```python
from build123d import *

# Parameters (mm, degrees)
EXTRUDE_1_DEPTH     = 22.5
SKETCH_2_R          = 8
CUT_EXTRUDE_1_DEPTH = 10
CUT_EXTRUDE_2_REACH = 62.26
SKETCH_3_R          = 5


with BuildPart() as part:
    # Эскиз1 → Бобышка-Вытянуть1 (new, symmetric)
    with BuildSketch(Plane(origin=(0, 0, 0), x_dir=(1, 0, 0), z_dir=(0, 1, 0))):
        Polygon((50, 0), (-50, 0), (-50, 30), (-20, 30), (-20, 45), (-8, 45), (-5, 42), (-5, 10), (5, 10), (5, 42), (8, 45), (20, 45), (20, 30), (50, 30), align=None)
    extrude(amount=EXTRUDE_1_DEPTH, both=True)

    # Эскиз2 → Вырез-Вытянуть1 (cut)
    with BuildSketch(Plane(origin=(0, 0, -30), x_dir=(-1, 0, 0), z_dir=(0, 0, -1))):
        with Locations((37.5, 0)):
            Circle(SKETCH_2_R)
    cut_extrude_1 = extrude(amount=-CUT_EXTRUDE_1_DEPTH, mode=Mode.SUBTRACT)

    # Эскиз3 → Вырез-Вытянуть2 (cut, up to next)
    with BuildSketch(Plane(origin=(0, 0, -20), x_dir=(-1, 0, 0), z_dir=(0, 0, -1)), mode=Mode.PRIVATE) as cut_extrude_2_sk1:
        with Locations((37.5, 0)):
            Circle(SKETCH_3_R)
    cut_extrude_2_tool1 = extrude(cut_extrude_2_sk1.sketch, amount=-CUT_EXTRUDE_2_REACH, mode=Mode.PRIVATE) & part.part
    cut_extrude_2 = cut_extrude_2_tool1.solids().sort_by_distance((-37.5, 0, -20))[0]
    add(cut_extrude_2, mode=Mode.SUBTRACT)

    # Зеркальное отражение1: Вырез-Вытянуть1, Вырез-Вытянуть2 across plane
    add(cut_extrude_1.mirror(Plane(origin=(0, 0, 0), x_dir=(0, 0, 1), z_dir=(1, 0, 0))), mode=Mode.SUBTRACT)
    add(cut_extrude_2.mirror(Plane(origin=(0, 0, 0), x_dir=(0, 0, 1), z_dir=(1, 0, 0))), mode=Mode.SUBTRACT)


solid = part.part
```
Source: CAD feature listing. Evaluate the final solid. Frame: model axes, mm. A direction names the side the tool comes from. Give positions to 0.01 mm unless a question says otherwise; leave off trailing zeros. Write each loop counter-clockwise with the first axis right and the second up, starting at its lowest first coordinate (ties: lowest second). Pieces come first, ordered by that corner, then holes.
1. Section query C-C (x = 37.5). Return the cut outline in (y, z), then the cut area to 3 significant figures.
2. Access query for faces 5 (the face through (6, 0, -43)), 6 (the face through (-29, 0, -30)), 7 (the face through (20, 0, -38)). Directions: +Z, -Z, +X, -X, +Y, -Y. A direction counts if a zero-diameter tool reaches every point of the face in a straight line with its end or side. Return the directions, or none.
3. Pull-direction query (Y, two-part tool) for faces 1 (the face through (41, 4, -20)), 2 (the face through (-50, 0, -15)), 3 (the face through (1, 22.5, -8)), 4 (the face through (31.151, -4.868, -25.07)); classes: +Y half, -Y half, draft (parallel to the pull), parting line (faces both ways), or undercut.
4. Section query D-D (z = -28.5). Return the cut outline in (x, y).
5. Section query A-A (z = -12). Return the cut outline in (x, y).
6. Section query B-B (y = 0). Count the separate pieces of the cut face and the enclosed holes in it, then the cut area to 3 significant figures.
7. First-contact query: pin 1 (17.5 mm diameter, centred on x = -37, y = 1.5, fed in from -Z); pin 2 (8 mm diameter, centred on x = 0, y = 8, fed in from -Z); pin 3 (7.5 mm diameter, centred on y = 10, z = -35.5, fed in from -X). Flat tips, straight axial feed; report the tip coordinate or a pass-through.
8. Material intervals for line 1 along X through (y, z) = (14.5, -14.5); line 2 along Y through (x, z) = (37, -23); line 3 along Y through (x, z) = (37.5, -8.5), sorted ascending.
Output values:
1. outline: (-22.5, -30) - (-8, -30) - (-8, -20) - (-5, -20) - (-5, 0) - (-22.5, 0) - close; (5, -20) - (8, -20) - (8, -30) - (22.5, -30) - (22.5, 0) - (5, 0) - close
1. area: 990 mm2
2. face 5: -Z, +Y, -Y
2. face 6: -Z, -X, +Y, -Y
2. face 7: -Z, +X, +Y, -Y
3. face 1: undercut
3. face 2: draft
3. face 3: +Y half
3. face 4: undercut
4. outline: (-50, -22.5) - (-5, -22.5) - (-5, 22.5) - (-50, 22.5) - close; (5, -22.5) - (50, -22.5) - (50, 22.5) - (5, 22.5) - close; hole circle Ø16 at (-37.5, 0); hole circle Ø16 at (37.5, 0)
5. outline: (-50, -22.5) - (-5, -22.5) - (-5, 22.5) - (-50, 22.5) - close; (5, -22.5) - (50, -22.5) - (50, 22.5) - (5, 22.5) - close; hole circle Ø10 at (-37.5, 0); hole circle Ø10 at (37.5, 0)
6. separate pieces: 3
6. enclosed holes: 0
6. area: 2,520 mm2
7. pin 1: stops at z = -30
7. pin 2: stops at z = -10
7. pin 3: stops at x = -20
8. line 1: x = -50 to -5, 5 to 50
8. line 2: y = -22.5 to -7.98, 7.98 to 22.5
8. line 3: y = -22.5 to -5, 5 to 22.5
